from build123d import *

# Parameters (mm, degrees)
F0_R     = 2.38125
F1_DEPTH = 7.9375
F2_R     = 3.175
F3_DEPTH = 4.7625
F4_R     = 7.14375
F5_DEPTH = 3.175
F6_R     = 6.35
F7_DEPTH = 3.96875


with BuildPart() as f1:
    # F0 (on Top) → F1 (new body, symmetric)
    with BuildSketch(Plane.XY):
        Circle(F0_R)
    extrude(amount=F1_DEPTH, both=True)

    # F2 (on Top) → F3 (join, symmetric)
    with BuildSketch(Plane.XY):
        Circle(F2_R)
    extrude(amount=F3_DEPTH, both=True)

    # F4 (on Top) → F5 (join, symmetric)
    with BuildSketch(Plane.XY):
        Circle(F4_R)
    extrude(amount=F5_DEPTH, both=True)

    # F6 (on Top) → F7 (join, symmetric)
    with BuildSketch(Plane.XY):
        Circle(F6_R)
    extrude(amount=F7_DEPTH, both=True)


solid = f1.part
Could you check a few things on this model? Use its own coordinates, in mm. A direction names the side the tool comes from. Give positions to 0.01 mm unless a question says otherwise; leave off trailing zeros. Order: outer loops, then holes, each group sorted by start corner. A loop starts at its lowest first (then second) coordinate and runs counter-clockwise, first axis right, second up. Notation, with made-up numbers: (-19.5, 87.25) - (15.5, 87.25) arc R5 ccw to (15.5, 93.25) - close; hole circle Ø9 at (-5.75, 7). An arc over 180 degrees is marked (long way). One line per item, written item: value. Start each with the question number.
1. Imagine slicing it at D-D on y = -4.5. List the corners of the cut face in (x, z) for me (3 decimals).
2. If I drill on probe 1 along Z at (x, y) = (0.5, 4); probe 2 along Z at (x, y) = (-5, 4.25) (3 decimals); probe 3 along X at (y, z) = (4, 2.25), over which ranges is the centre line in solid material (lowest first)?
3. For P1, Ø2, axis at x = -4.5, z = -2.5, coming from the +Y side; P2, Ø5, axis at x = 4.5, y = 4, coming from the -Z side; P3, Ø8, axis at x = 5.5, z = -3, coming from the -Y side, each with a flat end and sliding along its axis, tell me the tip position at first contact or that it passes through.
4. Imagine slicing it at C-C on z = 3.75. List the corners of the cut face in (x, y) for me.
5. For faces 1 (the face through (-6, -3, 3.175)), 2 (the face through (-7.137, 0.314, 0.044)), 3 (the face through (-6, -3, -3.175)), which set-ups out of +Z, -Z, +X, -X, +Y, -Y let a thin tool reach every point of the face, with its end or its side?
Values:
1. outline: (-5.548, -3.175) - (-4.48, -3.175) - (-4.48, -3.969) - (4.48, -3.969) - (4.48, -3.175) - (5.548, -3.175) - (5.548, 3.175) - (4.48, 3.175) - (4.48, 3.969) - (-4.48, 3.969) - (-4.48, 3.175) - (-5.548, 3.175) - close
2. probe 1: -3.97 to 3.97
2. probe 2: -3.175 to 3.175
2. probe 3: -5.92 to 5.92
3. P1: y = 6.23
3. P2: z = -3.97
3. P3: y = -6.98
4. outline: circle Ø12.7 at (0, 0)
5. face 1: +Z
5. face 2: +Z, -Z
5. face 3: -Z
